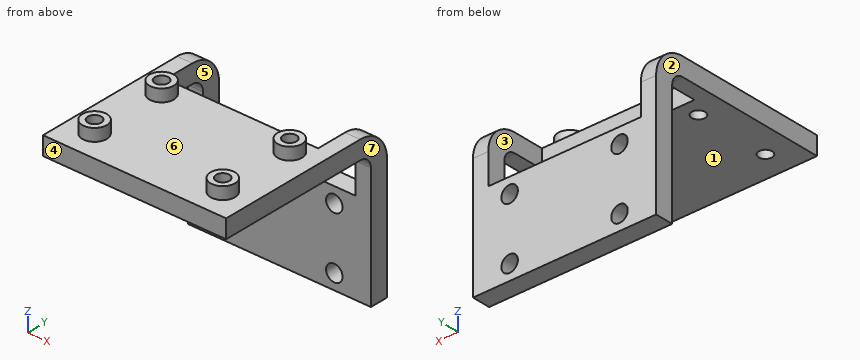
```python
from build123d import *

# Parameters (mm, degrees)
SKETCH2_W           = 30
SKETCH2_H           = 30
BOSS_EXTRUDE1_DEPTH = 3
SKETCH4_R           = 2
BOSS_EXTRUDE2_DEPTH = 2
SKETCH5_R           = 1.1
CUT_EXTRUDE1_DEPTH  = 12
SKETCH6_W           = 25
SKETCH6_H           = 7
CUT_EXTRUDE2_DEPTH  = 3
SKETCH9_W           = 30
SKETCH9_H           = 3
BOSS_EXTRUDE3_DEPTH = 22
SKETCH10_W          = 25
SKETCH10_H          = 3
CUT_EXTRUDE3_DEPTH  = 10
FILLET1_R           = 2
FILLET2_R           = 5
SKETCH11_R          = 1.35
CUT_EXTRUDE4_DEPTH  = 10


with BuildPart() as part:
    # Sketch2 → Boss-Extrude1 (new body)
    with BuildSketch(Plane.XY):
        Rectangle(SKETCH2_W, SKETCH2_H)
    extrude(amount=BOSS_EXTRUDE1_DEPTH)

    # Sketch4 → Boss-Extrude2 (add)
    with BuildSketch(Plane.XY.offset(3)):
        with Locations((-10.5, 2)):
            Circle(SKETCH4_R)
        with Locations((10.5, 2)):
            Circle(SKETCH4_R)
        with Locations((10.5, -10.5)):
            Circle(SKETCH4_R)
        with Locations((-10.5, -10.5)):
            Circle(SKETCH4_R)
    extrude(amount=BOSS_EXTRUDE2_DEPTH)

    # Sketch5 → Cut-Extrude1 (cut)
    with BuildSketch(Plane.XY.offset(5)):
        with Locations((10.5, 2)):
            Circle(SKETCH5_R)
        with Locations((-10.5, 2)):
            Circle(SKETCH5_R)
        with Locations((-10.5, -10.5)):
            Circle(SKETCH5_R)
        with Locations((10.5, -10.5)):
            Circle(SKETCH5_R)
    extrude(amount=-CUT_EXTRUDE1_DEPTH, mode=Mode.SUBTRACT)

    # Sketch6 → Cut-Extrude2 (cut)
    with BuildSketch(Plane.XY.offset(3)):
        with Locations((0, 8.5)):
            Rectangle(SKETCH6_W, SKETCH6_H)
    extrude(amount=-CUT_EXTRUDE2_DEPTH, mode=Mode.SUBTRACT)

    # Sketch9 → Boss-Extrude3 (add)
    with BuildSketch(Plane(origin=(0, 0, 0), x_dir=(-1, 0, 0), z_dir=(0, 0, -1))):
        with Locations((0, 13.5)):
            Rectangle(SKETCH9_W, SKETCH9_H)
    extrude(amount=BOSS_EXTRUDE3_DEPTH)

    # Sketch10 → Cut-Extrude3 (cut)
    with BuildSketch(Plane.XY.offset(3)):
        with Locations((0, 13.5)):
            Rectangle(SKETCH10_W, SKETCH10_H)
    extrude(amount=-CUT_EXTRUDE3_DEPTH, mode=Mode.SUBTRACT)

    # Fillet1
    fillet1_edges = [part.edges().sort_by_distance(p)[0] for p in [
        (-13.75, 12, 0),
        (13.75, 12, 0),
    ]]
    fillet(fillet1_edges, radius=FILLET1_R)

    # Fillet2
    fillet2_edges = [part.edges().sort_by_distance(p)[0] for p in [
        (-13.75, 15, 3),
        (13.75, 15, 3),
    ]]
    fillet(fillet2_edges, radius=FILLET2_R)

    # Sketch11 → Cut-Extrude4 (cut)
    with BuildSketch(Plane(origin=(0, 15, 0), x_dir=(1, 0, 0), z_dir=(0, 1, 0))):
        with Locations(Location((-9, 19.5, 0), (0, 0, 270))):
            Circle(SKETCH11_R)
        with Locations(Location((9, 19.5, 0), (0, 0, 270))):
            Circle(SKETCH11_R)
        with Locations(Location((-9, 9.5, 0), (0, 0, 270))):
            Circle(SKETCH11_R)
        with Locations(Location((9, 9.5, 0), (0, 0, 270))):
            Circle(SKETCH11_R)
    extrude(amount=-CUT_EXTRUDE4_DEPTH, mode=Mode.SUBTRACT)


solid = part.part
```
Read the model definition and answer for the solid it produces. Units are mm, in the model's axes. Face numbers are marked on the shaded views. A direction names the side the tool comes from. Coordinates: 2 decimals unless noted, no trailing zeros. Write each loop counter-clockwise with the first axis right and the second up, starting at its lowest first coordinate (ties: lowest second). Pieces come first, ordered by that corner, then holes. Notation, with made-up numbers: (57, 74) -> (88, 74) arc R14 cw to (88, 88) -> close; hole circle Ø5 at (-19.5, -12.5). An arc over 180 degrees is marked (long way). Answer as a JSON object with one key per item and string values.
Q1. The part is cut by section B-B on y = 9.5. Give the vertices of the cut face in (x, z).
The answers:
{"outline": "(-15, 0) -> (-12.5, 0) -> (-12.5, 3) -> (-15, 3) -> close; (12.5, 0) -> (15, 0) -> (15, 3) -> (12.5, 3) -> close"}
Q2. The part is cut by section A-A on x = 2.25. Give the vertices of the cut face in (y, z), then the cut area to 3 significant figures.
The answers:
{"outline": "(-15, 0) -> (5, 0) -> (5, 3) -> (-15, 3) -> close; (12, -22) -> (15, -22) -> (15, -7) -> (12, -7) -> close", "area": "105 mm2"}
Q3. The part is cut by section D-D on y = 2. Give the vertices of the cut face in (x, z), then the cut area to 3 significant figures.
The answers:
{"outline": "(-15, 0) -> (-11.6, 0) -> (-11.6, 5) -> (-12.5, 5) -> (-12.5, 3) -> (-15, 3) -> close; (-9.4, 0) -> (9.4, 0) -> (9.4, 5) -> (8.5, 5) -> (8.5, 3) -> (-8.5, 3) -> (-8.5, 5) -> (-9.4, 5) -> close; (11.6, 0) -> (15, 0) -> (15, 3) -> (12.5, 3) -> (12.5, 5) -> (11.6, 5) -> close", "area": "84.0 mm2"}
Q4. Consider line 1 (Y direction, x = 10.5, z = 2.45); line 2 (X direction, y = 13.1, z = -9.5); line 3 (Z direction, x = 6.75, y = -6.75). Determine where each line is inside the solid, lowest interval first. Write a range as [from, to].
The answers:
{"line 1": "y = [-15, -11.6], [-9.4, 0.9], [3.1, 5]", "line 2": "x = [-15, -10.35], [-7.65, 7.65], [10.35, 15]", "line 3": "z = [0, 3]"}
Q5. Flat-ended cylindrical pins translate along their axes: pin 1 Ø7.5 at (x, y) = (-5, -6) entering from -Z; pin 2 Ø8 at (x, y) = (-1, -10) entering from +Z; pin 3 Ø2.5 at (x, z) = (-0.5, 1.5) entering from +Y. Find the tip coordinate at first contact, or state that the pin passes through.
The answers:
{"pin 1": "stops at z = 0", "pin 2": "stops at z = 3", "pin 3": "stops at y = 5"}
Q6. The part is cut by section C-C on z = -9.5. Give the vertices of the cut face in (x, y), then the cut area to 3 significant figures.
The answers:
{"outline": "(-15, 12) -> (-10.35, 12) -> (-10.35, 15) -> (-15, 15) -> close; (-7.65, 12) -> (7.65, 12) -> (7.65, 15) -> (-7.65, 15) -> close; (10.35, 12) -> (15, 12) -> (15, 15) -> (10.35, 15) -> close", "area": "73.8 mm2"}
Q7. A tool of negligible diameter and unlimited length cuts with its end or side. For the marked faces 1, 2 and 3, from which of +Z, -Z, +X, -X, +Y, -Y can it reach the whole face along a straight path? Write none if from no direction.
The answers:
{"face 1": "-Z, +X, -X, -Y", "face 2": "+Z, -Z, -X, +Y, -Y", "face 3": "+Z, +Y"}
Q8. Determine the mould class of the marked faces 4, 5, 6 and 7 for opening direction X: pulls with the +X half, pulls with the -X half, needs draft (parallel to the pull), parting line crosses it, or undercut.
The answers:
{"face 4": "needs draft", "face 5": "undercut", "face 6": "undercut", "face 7": "pulls with the +X half"}
